Print and shaded views of the part. All mm, measured from the part's lowest x, y and z. A direction names the side the tool comes from. Coordinates: 2 decimals unless noted, no trailing zeros. Order: outer loops, then holes, each group sorted by start corner. A loop starts at its lowest first (then second) coordinate and runs counter-clockwise, first axis right, second up. Notation, with made-up numbers: (21.25, 15) - (59.25, 15) arc R13 ccw to (59.25, 37) - close; hole circle Ø10 at (-30.75, 62.5). An arc over 180 degrees is marked (long way). Write each question's results on one line, items separated by ' | '.
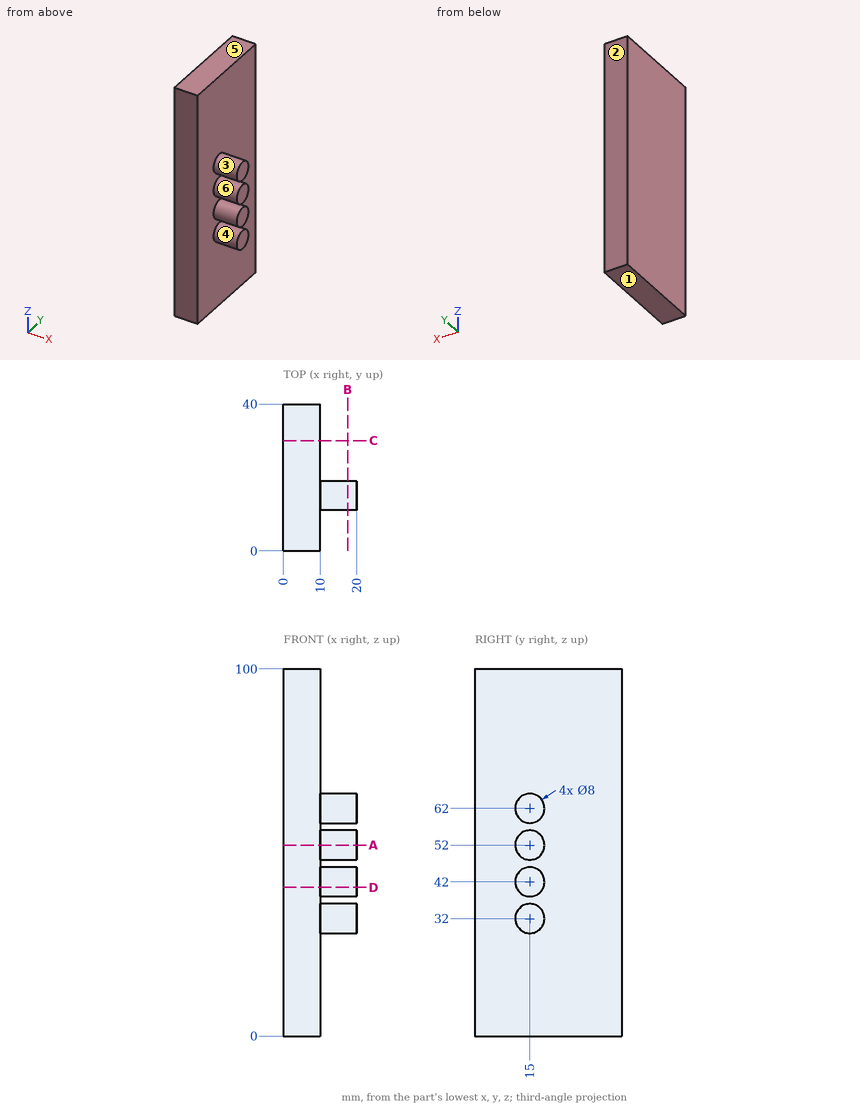
1. Band-saw the part on B-B on x = 17.5. Give the cut face in (y, z).
Solved:
outline: circle Ø8 at (15, 32); circle Ø8 at (15, 42); circle Ø8 at (15, 52); circle Ø8 at (15, 62)
2. Probe line 1 (Z direction, x = 13.75, y = 17.5); line 2 (Z direction, x = 18.5, y = 11.5); line 3 (X direction, y = 26, z = 86). List the from-to ranges inside material, lowest first.
Solved:
line 1: z = 28.88 to 35.12, 38.88 to 45.12, 48.88 to 55.12, 58.88 to 65.12 | line 2: z = 30.06 to 33.94, 40.06 to 43.94, 50.06 to 53.94, 60.06 to 63.94 | line 3: x = 0 to 10
3. Drop flat-ended pins along their axis: pin 1 Ø4 at (y, z) = (14.5, 82.5) entering from -X; pin 2 Ø3 at (y, z) = (4, 30.5) entering from +X. Give the stop position or say it passes through.
Solved:
pin 1: stops at x = 0 | pin 2: stops at x = 10
4. Band-saw the part on D-D on z = 40.5. Give the cut face in (x, y), then the cut area to 3 significant figures.
Solved:
outline: (0, 0) - (10, 0) - (10, 11.29) - (20, 11.29) - (20, 18.71) - (10, 18.71) - (10, 40) - (0, 40) - close | area: 474 mm2
5. Band-saw the part on A-A on z = 52. Give the cut face in (x, y), then the cut area to 3 significant figures.
Solved:
outline: (0, 0) - (10, 0) - (10, 11) - (20, 11) - (20, 19) - (10, 19) - (10, 40) - (0, 40) - close | area: 480 mm2
6. Band-saw the part on C-C on y = 30. Give the cut face in (x, z), then the cut area to 3 significant figures.
Solved:
outline: (0, 0) - (10, 0) - (10, 100) - (0, 100) - close | area: 1,000 mm2
7. Tool access for the marked faces 5 and 6: list every direction of +Z, -Z, +X, -X, +Y, -Y with a clear straight run to the whole face (end or side of a thin tool).
Solved:
face 5: +Z, +X, -X, +Y, -Y | face 6: +X
8. Two-plate mould, pull along Z, no slides. Class the marked faces 1, 2, 3 and 4: +Z half, -Z half, draft (parallel to the pull), parting line (faces both ways), or undercut.
Solved:
face 1: -Z half | face 2: draft | face 3: undercut | face 4: undercut
